from build123d import *

# Parameters (mm, degrees)
BOSS_EXTRUDE1_DEPTH = 1.5875
CUT_EXTRUDE1_DEPTH  = 159.638836079


with BuildPart() as part:
    # Sketch1 → Boss-Extrude1 (new body)
    with BuildSketch(Plane(origin=(0, 0, 0), x_dir=(1, 0, 0), z_dir=(0, 1, 0))):
        Polygon((-150.8125, 25.4), (-153.9875, 25.4), (-153.9875, -25.4), (-150.8125, -25.4), (-150.8125, -38.1), (150.8125, -38.1), (150.8125, -25.4), (153.9875, -25.4), (153.9875, 25.4), (150.8125, 25.4), (150.8125, 38.1), (-150.8125, 38.1), align=None)
    extrude(amount=BOSS_EXTRUDE1_DEPTH)

    # Sketch2 → Cut-Extrude1 (cut, through all)
    with BuildSketch(Plane(origin=(0, 1.5875, 0), x_dir=(1, 0, 0), z_dir=(0, 1, 0))):
        with BuildLine():
            Line((-138.1125, 19.05), (-138.1125, -13.638858994))
            ThreePointArc((-138.1125, -13.638858994), (-135.664170115, -18.648796151), (-130.207155019, -19.795432878))
            Line((-130.207155019, -19.795432878), (28.889358139, 20.397370446))
            ThreePointArc((28.889358139, 20.397370446), (30.78780332, 23.173465256), (28.267220147, 25.4))
            Line((28.267220147, 25.4), (-131.7625, 25.4))
            ThreePointArc((-131.7625, 25.4), (-136.252628061, 23.540128061), (-138.1125, 19.05))
        make_face()
        with BuildLine():
            Line((-28.267220147, -25.4), (131.7625, -25.4))
            ThreePointArc((131.7625, -25.4), (136.252628061, -23.540128061), (138.1125, -19.05))
            Line((138.1125, -19.05), (138.1125, 13.638858994))
            ThreePointArc((138.1125, 13.638858994), (135.664170115, 18.648796151), (130.207155019, 19.795432878))
            Line((130.207155019, 19.795432878), (-28.889358139, -20.397370446))
            ThreePointArc((-28.889358139, -20.397370446), (-30.78780332, -23.173465256), (-28.267220147, -25.4))
        make_face()
    extrude(amount=-CUT_EXTRUDE1_DEPTH, mode=Mode.SUBTRACT)


solid = part.part
Verification items for the finished model (mm, model axes). A direction names the side the tool comes from. Round coordinates to 2 decimals unless told otherwise and drop trailing zeros. Order: outer loops, then holes, each group sorted by start corner. A loop starts at its lowest first (then second) coordinate and runs counter-clockwise, first axis right, second up.
1. Section check A-A on x = -56.5. Record the cut outline in (y, z).
Final values:
outline: (0, -38.1) - (1.59, -38.1) - (1.59, -25.4) - (0, -25.4) - close; (0, 1.17) - (1.59, 1.17) - (1.59, 38.1) - (0, 38.1) - close
2. Thickness scan on L1, parallel to Z at x = 0, y = 1.5; L2, parallel to Z at x = -11.5, y = 0.2; L3, parallel to Z at x = -118.5, y = 0.3. Record the ranges inside material, lowest first.
Final values:
L1: z = -38.1 to -25.4, -13.1 to 13.1, 25.4 to 38.1
L2: z = -38.1 to -25.4, -10.19 to 16, 25.4 to 38.1
L3: z = -38.1 to -25.4, 16.84 to 38.1
3. Section check D-D on x = -23. Record the cut outline in (y, z).
Final values:
outline: (0, -38.1) - (1.59, -38.1) - (1.59, -25.4) - (0, -25.4) - close; (0, -7.29) - (1.59, -7.29) - (1.59, 18.91) - (0, 18.91) - close; (0, 25.4) - (1.59, 25.4) - (1.59, 38.1) - (0, 38.1) - close
4. Section check C-C on z = 2.5. Record the cut outline in (x, y), then the cut area to 3 significant figures.
Final values:
outline: (-153.99, 0) - (-138.11, 0) - (-138.11, 1.59) - (-153.99, 1.59) - close; (-61.75, 0) - (41.95, 0) - (41.95, 1.59) - (-61.75, 1.59) - close; (138.11, 0) - (153.99, 0) - (153.99, 1.59) - (138.11, 1.59) - close
area: 215 mm2
5. Go/stop test with flat-tipped pins: P1, Ø0.8, axis at y = 0.5, z = 31.5, coming from the -X side; P2, Ø4, axis at x = 115, z = -13, coming from the -Y side; P3, Ø0.5, axis at y = 0.5, z = -31.5, coming from the +X side; P4, Ø0.8, axis at x = -152.5, y = 1, coming from the -Z side. Record where each tip stops, or that it passes through.
Final values:
P1: stops at x = -150.81
P2: passes through
P3: stops at x = 150.81
P4: stops at z = -25.4
6. Release check for a two-part mould opening along X. For faces 3 (the flat face through (-2, 1.588, -1)), 4 (the cylindrical face through (-136.2, 0.8, -23.59)), 5 (the cylindrical face through (135.728, 0.805, -18.599)) record: +X half, -X half, draft (parallel to the pull), parting line (faces both ways), or undercut.
Final values:
face 3: draft
face 4: undercut
face 5: undercut
7. Access from +Z, -Z, +X, -X, +Y, -Y to the whole of each face (thin tool, end or side, straight path). Record for faces 1 (the flat face through (-2, 0, -1)), 2 (the cylindrical face through (136.2, 0.8, 23.59)).
Final values:
face 1: +Z, -Z, +X, -X, -Y
face 2: +Y, -Y
8. Section check B-B on y = 1.1. Record the cut outline in (x, z), then the cut area to 3 significant figures.
Final values:
outline: (-153.99, -25.4) - (-150.81, -25.4) - (-150.81, -38.1) - (150.81, -38.1) - (150.81, -25.4) - (153.99, -25.4) - (153.99, 25.4) - (150.81, 25.4) - (150.81, 38.1) - (-150.81, 38.1) - (-150.81, 25.4) - (-153.99, 25.4) - close; hole (-138.11, -19.05) arc R6.35 ccw to (-131.76, -25.4) - (28.27, -25.4) arc R2.54 ccw to (28.89, -20.4) - (-130.21, 19.8) arc R6.35 ccw to (-138.11, 13.64) - close; hole (-28.89, 20.4) - (130.21, -19.8) arc R6.35 ccw to (138.11, -13.64) - (138.11, 19.05) arc R6.35 ccw to (131.76, 25.4) - (-28.27, 25.4) arc R2.54 ccw to start
area: 14,600 mm2
